from build123d import *

# Parameters (mm, degrees)
F1_DEPTH       = 12
F4_D           = 4
F4_DEPTH       = 5
F4_CSINK_D     = 8
F4_CSINK_ANGLE = 90
F4_TIP         = 1.2017212381
F3_R           = 4
F5_DEPTH       = 26.0010001


with BuildPart() as f1:
    # F0 (on Top) → F1 (new body)
    with BuildSketch(Plane.XY):
        with BuildLine():
            Line((-25, 0), (0, 0))
            Line((0, 0), (0, 26))
            ThreePointArc((0, 26), (0.5857864376, 27.4142135624), (2, 28))
            Line((2, 28), (10, 28))
            Line((10, 28), (10, 29))
            ThreePointArc((10, 29), (9.4142135624, 30.4142135624), (8, 31))
            Line((8, 31), (-3, 31))
            add(Edge.make_bspline(
                [(-3, 31), (-8.7686244949, 31), (-0.6718204217, 6.9665904818), (-22.256677699, 5.1130097266)],
                knots=[0, 0, 0, 0, 32.7453784414, 32.7453784414, 32.7453784414, 32.7453784414], degree=3))
            ThreePointArc((-22.256677699, 5.1130097266), (-24.2102073542, 4.1525526681), (-25, 2.1240104696))
            Line((-25, 2.1240104696), (-25, 0))
        make_face()
    extrude(amount=F1_DEPTH)

    # F4
    with Locations(Plane(origin=(0, 5, 0), x_dir=(1, 0, 0), z_dir=(0, 1, 0))):
        with Locations((-19, -6)):
            CounterSinkHole(F4_D / 2, F4_CSINK_D / 2, depth=F4_DEPTH, counter_sink_angle=F4_CSINK_ANGLE)
            with Locations((0, 0, -(F4_DEPTH + F4_TIP / 2))):  # 118° drill point
                Cone(0, F4_D / 2, F4_TIP, mode=Mode.SUBTRACT)

    # F3 (on offset) → F5 (cut, through all)
    with BuildSketch(Plane.XZ.offset(-5)):
        with Locations((-19, 6)):
            Circle(F3_R)
    extrude(amount=-F5_DEPTH, mode=Mode.SUBTRACT)


solid = f1.part
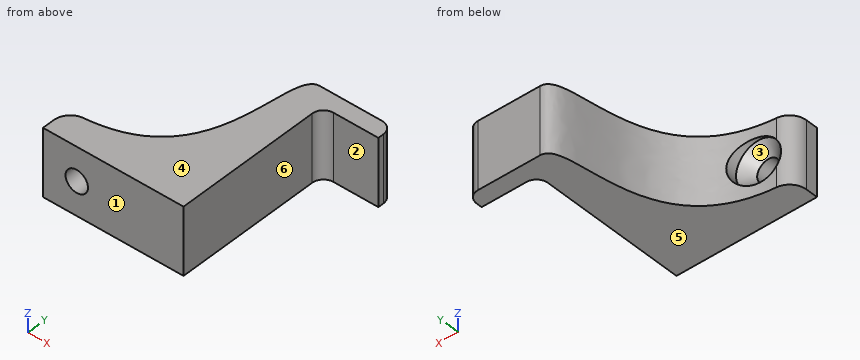
The model under review builds one solid part; all positions refer to its coordinate system, in mm. Face numbers are marked on the shaded views. A direction names the side the tool comes from. Coordinates: 2 decimals unless noted, no trailing zeros. Order: outer loops, then holes, each group sorted by start corner. A loop starts at its lowest first (then second) coordinate and runs counter-clockwise, first axis right, second up. Notation, with made-up numbers: (63, 79.5) -> (106, 79.5) arc R29 cw to (106, 117.5) -> close; hole circle Ø10 at (-20.75, 44). An arc over 180 degrees is marked (long way). Answer in a Markdown table with one row per item.
(1) Wall thickness on line 1 along Z through (x, y) = (-19, 1.35); line 2 along X through (y, z) = (5.9, 6); line 3 along Z through (x, y) = (-19, 5): over which ranges is each line inside the solid? List them lowest first.
Answers:
| item | result |
|---|---|
| line 1 | 0 to 4, 8 to 12 |
| line 2 | -15 to 0 |
| line 3 | 0 to 2, 10 to 12 |
(2) Machinability: for the marked faces 1 and 2, which of the approach directions +Z, -Z, +X, -X, +Y, -Y give a long, thin tool a straight path to every point of the face, cutting with its end or side? Answer none if there is none.
Answers:
| item | result |
|---|---|
| face 1 | +Z, -Z, +X, -X, -Y |
| face 2 | +Z, -Z, +X, -Y |
(3) Consider section A-A (x = 4). Write out the cut boundary in (y, z).
Answers:
| item | result |
|---|---|
| outline | (28, 0) -> (31, 0) -> (31, 12) -> (28, 12) -> close |
(4) Insertion check: pin 1 (1.5 mm diameter, centred on y = 16.5, z = 1.5, fed in from +X); pin 2 (6 mm diameter, centred on y = 11.5, z = 6.5, fed in from -X); pin 3 (2.5 mm diameter, centred on x = 4, z = 3.5, fed in from -Y); pin 4 (12 mm diameter, centred on x = -18, y = 18, fed in from +Z). Each pin has a flat end and moves straight along its axis. Give the tip position at first contact, or say it passes through.
Answers:
| item | result |
|---|---|
| pin 1 | x = 0 |
| pin 2 | x = -12.54 |
| pin 3 | y = 28 |
| pin 4 | through |
(5) The part is to be moulded in two halves that separate along Z. For the marked faces 3, 4, 5 and 6, say which applies: +Z half, -Z half, draft (parallel to the pull), parting line (faces both ways), or undercut.
Answers:
| item | result |
|---|---|
| face 3 | undercut |
| face 4 | +Z half |
| face 5 | -Z half |
| face 6 | draft |
